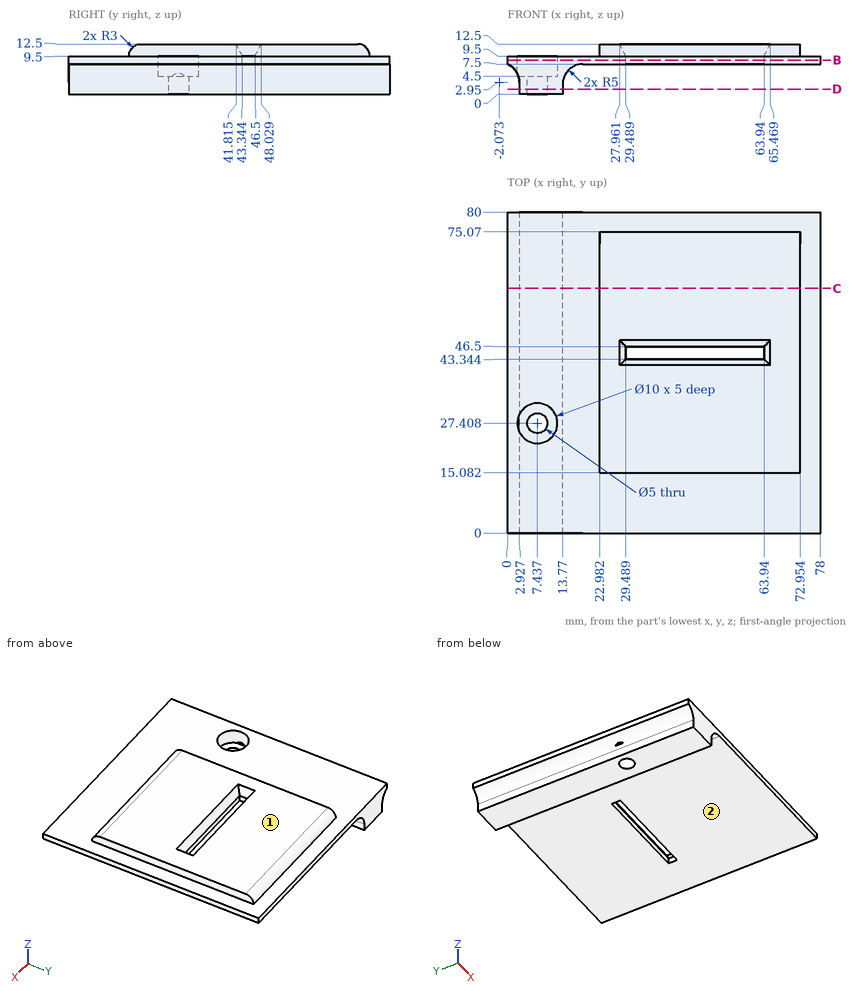
Input: dimensioned drawing with shaded views. Units: mm. Origin: part minimum x, y, z. A direction names the side the tool comes from. Round coordinates to 2 decimals unless told otherwise and drop trailing zeros. Order: outer loops, then holes, each group sorted by start corner. A loop starts at its lowest first (then second) coordinate and runs counter-clockwise, first axis right, second up. Notation, with made-up numbers: (75, 25.5) -> (85, 25.5) arc R26 cw to (85, 63.5) -> close; hole circle Ø7 at (-9, 18). An arc over 180 degrees is marked (long way). One line per item, written item: value. Start each with the question number.
Q1. Section query B-B (z = 8.5). Return the cut outline in (x, y), plus the area to 3 significant figures.
Q2. Section query D-D (z = 1.25). Return the cut outline in (x, y).
Q3. Access query for the marked faces 1 and 2. Directions: +Z, -Z, +X, -X, +Y, -Y. A direction counts if a zero-diameter tool reaches every point of the face in a straight line with its end or side. Return the directions, or none.
Q4. Section query C-C (y = 61). Return the cut outline in (x, z).
Q5. Pin query (flat end, axial travel): pin 1 (0.9 mm diameter, centred on y = 34.5, z = 2, fed in from -X); pin 2 (0.9 mm diameter, centred on y = 41.5, z = 10.5, fed in from +X); pin 3 (2 mm diameter, centred on x = 11.5, y = 48.5, fed in from +Z). Return the tip coordinate at first contact, or that it passes through.
Q6. Material intervals for probe 1 along Z at (x, y) = (52, 70); probe 2 along X at (y, z) = (25, 10.5); probe 3 along Y at (x, z) = (59, 8), sorted ascending.
Findings below:
1. outline: (0, 0) -> (78, 0) -> (78, 80) -> (0, 80) -> close; hole circle Ø10 at (7.44, 27.41); hole (29.49, 43.34) -> (63.94, 43.34) -> (63.94, 46.5) -> (29.49, 46.5) -> close
1. area: 6,050 mm²
2. outline: (2.93, 0) -> (13.77, 0) -> (13.77, 80) -> (2.93, 80) -> close; hole circle Ø5 at (7.44, 27.41)
3. face 1: +Z, +X, -X, +Y, -Y
3. face 2: -Z, +X, +Y, -Y
4. outline: (0, 7.5) arc R5 cw to (2.93, 2.95) -> (2.93, 0) -> (13.77, 0) -> (13.77, 2.5) arc R5 cw to (18.77, 7.5) -> (78, 7.5) -> (78, 9.5) -> (72.95, 9.5) -> (72.95, 12.5) -> (22.98, 12.5) -> (22.98, 9.5) -> (0, 9.5) -> close
5. pin 1: x = 2.93
5. pin 2: x = 72.95
5. pin 3: z = 9.5
6. probe 1: 7.5 to 12.5
6. probe 2: 22.98 to 72.95
6. probe 3: 0 to 43.34, 46.5 to 80
